Model file for the job. Use its own axes, mm. Face numbers are marked on the shaded views. A direction names the side the tool comes from. Round coordinates to 2 decimals unless told otherwise and drop trailing zeros. Order: outer loops, then holes, each group sorted by start corner. A loop starts at its lowest first (then second) coordinate and runs counter-clockwise, first axis right, second up. Notation, with made-up numbers: (6, -16.5) -> (22, -16.5) arc R24 ccw to (22, 19.5) -> close; hole circle Ø8 at (19, 17.5). An arc over 180 degrees is marked (long way). Use CSV: the item, a comma, the result in double quotes.
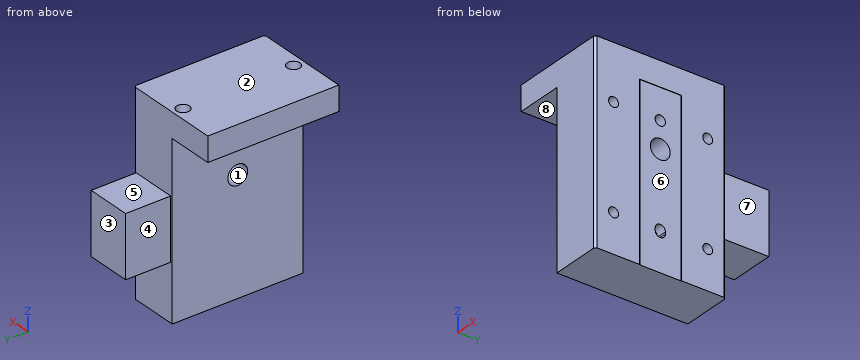
```python
from build123d import *

# Parameters (mm, degrees)
BASE_EXTRUDE_DEPTH               = 12
BOSS_EXTRUDE1_DEPTH              = 84
BOSS_EXTRUDE3_DEPTH              = 12
F_9_7_DIAMETER_HOLE1_D           = 9.7
F_10_32_TAPPED_HOLE1_D           = 4.0386
F_10_32_TAPPED_HOLE1_DEPTH       = 12.8624
F_10_32_TAPPED_HOLE1_CBORE_D     = 4.826
F_10_32_TAPPED_HOLE1_CBORE_DEPTH = 8.9
F_10_32_TAPPED_HOLE1_TIP         = 1.213317848
F_1_4_20_TAPPED_HOLE1_D          = 6.35
F_1_4_20_TAPPED_HOLE1_DEPTH      = 12
CUT_EXTRUDE1_DEPTH               = 5
HOLE1_D                          = 5
HOLE1_DEPTH                      = 5
SKETCH14_W                       = 22.1254
SKETCH14_H                       = 30
BOSS_EXTRUDE2_DEPTH              = 22
CHAMFER1_SIZE                    = 1


with BuildPart() as part:
    # Sketch1 → Base-Extrude (new body)
    with BuildSketch(Plane.XY.offset(-1312.73981158)):
        Polygon((-10.1873, 32), (37.3127, 32), (37.3127, 10.2), (37.1127, 10), (37.1127, -10), (37.3127, -10.2), (37.3127, -32), (-10.1873, -32), align=None)
    extrude(amount=BASE_EXTRUDE_DEPTH)

    # Sketch3 → Boss-Extrude1 (add)
    with BuildSketch(Plane(origin=(0, 0, -1312.73981158), x_dir=(-1, 0, 0), z_dir=(0, 0, -1))):
        Polygon((-37.3127, 10.2), (-37.3127, 32), (-12.6873, 32), (-12.6873, -32), (-37.3127, -32), (-37.3127, -10.2), (-37.1127, -10), (-37.1127, 10), align=None)
    extrude(amount=BOSS_EXTRUDE1_DEPTH)

    # Sketch15 → Boss-Extrude3 (add)
    with BuildSketch(Plane.XY.offset(-1300.73981158)):
        Polygon((37.1127, -10), (37.1127, 10), (37.3127, 10.2), (37.3127, -10.2), align=None)
    extrude(amount=-BOSS_EXTRUDE3_DEPTH)

    # 9.7 Diameter Hole1 (through all)
    with Locations(Plane(origin=(37.1127, 0, 0), x_dir=(0, 0, -1), z_dir=(1, 0, 0))):
        with Locations((1340.73981158, 0)):
            Hole(F_9_7_DIAMETER_HOLE1_D / 2)

    # #10-32 Tapped Hole1
    with Locations(Plane(origin=(37.3127, 0, 0), x_dir=(0, 0, -1), z_dir=(1, 0, 0))):
        with Locations((1327.73981158, 23), (1377.73981158, 23), (1327.73981158, -23), (1377.73981158, -23)):
            CounterBoreHole(F_10_32_TAPPED_HOLE1_D / 2, F_10_32_TAPPED_HOLE1_CBORE_D / 2, F_10_32_TAPPED_HOLE1_CBORE_DEPTH, depth=F_10_32_TAPPED_HOLE1_DEPTH)
            with Locations((0, 0, -(F_10_32_TAPPED_HOLE1_DEPTH + F_10_32_TAPPED_HOLE1_TIP / 2))):  # 118° drill point
                Cone(0, F_10_32_TAPPED_HOLE1_D / 2, F_10_32_TAPPED_HOLE1_TIP, mode=Mode.SUBTRACT)

    # 1/4-20 Tapped Hole1
    with Locations(Plane.XY.offset(-1300.73981158)):
        with Locations((12.3127, 27), (12.3127, -27)):
            Hole(F_1_4_20_TAPPED_HOLE1_D / 2, depth=F_1_4_20_TAPPED_HOLE1_DEPTH)

    # Sketch11 → Cut-Extrude1 (cut)
    with BuildSketch(Plane(origin=(37.1127, 0, 0), x_dir=(0, 0, -1), z_dir=(1, 0, 0))):
        with BuildLine():
            Line((1377.23981158, 2.5), (1378.23981158, 2.5))
            ThreePointArc((1378.23981158, 2.5), (1380.73981158, 0), (1378.23981158, -2.5))
            Line((1378.23981158, -2.5), (1377.23981158, -2.5))
            ThreePointArc((1377.23981158, -2.5), (1374.73981158, 0), (1377.23981158, 2.5))
        make_face()
    extrude(amount=-CUT_EXTRUDE1_DEPTH, mode=Mode.SUBTRACT)

    # Hole1
    with Locations(Plane(origin=(37.1127, 0, 0), x_dir=(0, 0, -1), z_dir=(1, 0, 0))):
        with Locations((1327.73981158, 0)):
            Hole(HOLE1_D / 2, depth=HOLE1_DEPTH)

    # Sketch14 → Boss-Extrude2 (add)
    with BuildSketch(Plane(origin=(0, 32, 0), x_dir=(-1, 0, 0), z_dir=(0, 1, 0))):
        with Locations((-24.75, -1354.23981158)):
            Rectangle(SKETCH14_W, SKETCH14_H)
    extrude(amount=BOSS_EXTRUDE2_DEPTH)

    # Chamfer1
    chamfer1_edges = [part.edges().sort_by_distance(p)[0] for p in [
        (37.3127, -32, -1348.73981158),
        (37.3127, 32, -1348.73981158),
    ]]
    chamfer(chamfer1_edges, length=CHAMFER1_SIZE)


solid = part.part
```
Q1. Mould opens along Y. For the marked faces 1, 2 and 3 say: +Y half, -Y half, draft (parallel to the pull), parting line (faces both ways), or undercut.
From the geometry:
face 1,"undercut"
face 2,"draft"
face 3,"+Y half"
Q2. Which spindle directions (+Z, -Z, +X, -X, +Y, -Y) get a long thin tool onto all of the face, cutting with end or side? Do the marked faces 4, 5, 6, 7 and 8. Say none if no direction does.
From the geometry:
face 4,"+Z, -Z, -X, +Y"
face 5,"+Z, +X, -X, +Y"
face 6,"-Z, +X"
face 7,"+Z, -Z, +X, +Y"
face 8,"-Z, -X, +Y, -Y"
Q3. Cut at B-B (z = -1337.5). Give the cut face in (x, y), plus the area to 3 significant figures.
From the geometry:
outline,"(12.69, -32) -> (36.31, -32) -> (37.31, -31) -> (37.31, -10.2) -> (37.11, -10) -> (37.11, -3.61) -> (12.69, -3.61) -> close; (12.69, 3.61) -> (37.11, 3.61) -> (37.11, 10) -> (37.31, 10.2) -> (37.31, 31) -> (36.31, 32) -> (12.69, 32) -> close"
area,"1,390 mm²"
Q4. Pin check, flat tips, straight feed: pin 1 (1.5 mm diameter, centred on x = 12, z = -1331, fed in from -Y); pin 2 (3.5 mm diameter, centred on y = 23, z = -1327.74, fed in from +X); pin 3 (7.5 mm diameter, centred on y = 23, z = -1377.74, fed in from -X); pin 4 (5.5 mm diameter, centred on y = -1, z = -1378.5, fed in from +X). Stop position of each tip, or through.
From the geometry:
pin 1,"stops at y = -32"
pin 2,"stops at x = 24.29"
pin 3,"stops at x = 12.69"
pin 4,"stops at x = 37.11"
Q5. Probe line 1 along Y through (x, z) = (-5, -1305.5); line 2 along X through (y, z) = (-24, -1324.5); line 3 along Z through (x, y) = (12, 2.5). List the from-to ranges inside material, lowest first.
From the geometry:
line 1,"y = -32 to 32"
line 2,"x = 12.69 to 37.31"
line 3,"z = -1312.74 to -1300.74"
Q6. Cut at C-C (z = -1320). Give the cut face in (x, y).
From the geometry:
outline,"(12.69, -32) -> (36.31, -32) -> (37.31, -31) -> (37.31, -10.2) -> (37.11, -10) -> (37.11, 10) -> (37.31, 10.2) -> (37.31, 31) -> (36.31, 32) -> (12.69, 32) -> close"
Q7. Cut at A-A (y = -27). Give the cut face in (x, z), plus the area to 3 significant figures.
From the geometry:
outline,"(-10.19, -1312.74) -> (9.14, -1312.74) -> (9.14, -1300.74) -> (-10.19, -1300.74) -> close; (12.69, -1396.74) -> (37.31, -1396.74) -> (37.31, -1300.74) -> (15.49, -1300.74) -> (15.49, -1312.74) -> (12.69, -1312.74) -> close"
area,"2,560 mm²"
Q8. Cut at D-D (y = -18). Give the cut face in (x, z), plus the area to 3 significant figures.
From the geometry:
outline,"(-10.19, -1312.74) -> (12.69, -1312.74) -> (12.69, -1396.74) -> (37.31, -1396.74) -> (37.31, -1300.74) -> (-10.19, -1300.74) -> close"
area,"2,640 mm²"
